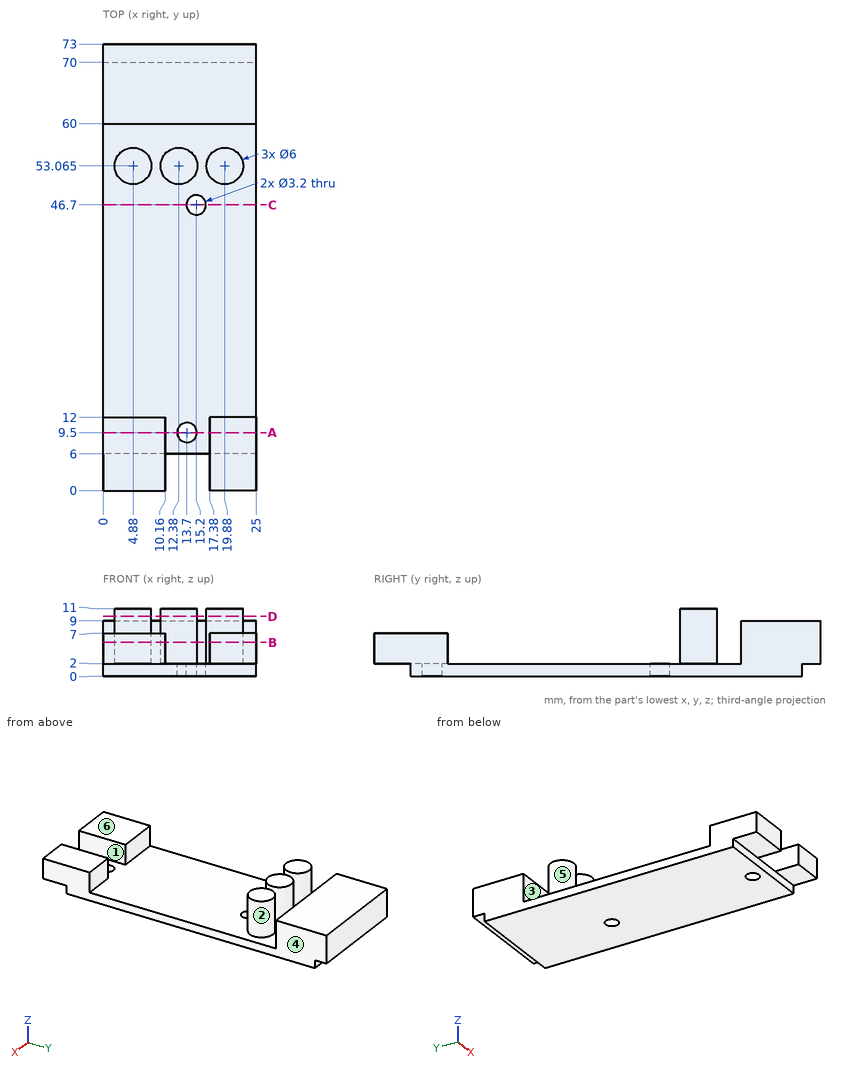
Study the drawing (mm; zero at the part's minimum x, y, z) and answer. A direction names the side the tool comes from. Give positions to 0.01 mm unless a question says otherwise; leave off trailing zeros. Write each loop counter-clockwise with the first axis right and the second up, starting at its lowest first coordinate (ties: lowest second). Pieces come first, ordered by that corner, then holes. Notation, with made-up numbers: (-26, -31) -> (0, -31) arc R19 cw to (0, -23) -> close; hole circle Ø7 at (75.25, 86). An arc over 180 degrees is marked (long way). Answer in a Markdown table with one row per item.
1) Each of these flat-tipped pins is pushed along its axis until it touches: pin 1 Ø1.5 at (x, z) = (12, 6) entering from -Y (1 decimal); pin 2 Ø3 at (x, z) = (3, 8) entering from -Y; pin 3 Ø1.5 at (x, z) = (18.5, 1) entering from -Y; pin 4 Ø2.5 at (x, y) = (21, 8) entering from +Z. Where does it stop, or does it pass through?
Results list:
| item | result |
|---|---|
| pin 1 | y = 50.1 |
| pin 2 | y = 0 |
| pin 3 | y = 6 |
| pin 4 | z = 7 |
2) Section D-D on z = 9.75 is taken. Give the vertices of the cut face in (x, y) (1 decimal).
Results list:
| item | result |
|---|---|
| outline | circle Ø6 at (4.9, 53.1); circle Ø6 at (12.4, 53.1); circle Ø6 at (19.9, 53.1) |
3) A tool of negligible diameter and unlimited length cuts with its end or side. For the marked faces 1, 2 and 3, from which of +Z, -Z, +X, -X, +Y, -Y can it reach the whole face along a straight path? Write none if from no direction.
Results list:
| item | result |
|---|---|
| face 1 | +Z, -Y |
| face 2 | +Z |
| face 3 | +Z, +X, -X |
4) Section B-B on z = 5.5 is taken. Give the vertices of the cut face in (x, y) (1 decimal), plus the area to 3 significant figures.
Results list:
| item | result |
|---|---|
| outline | (0, 0) -> (10.2, 0) -> (10.2, 12) -> (0, 12) -> close; (0, 60) -> (25, 60) -> (25, 73) -> (0, 73) -> close; circle Ø6 at (4.9, 53.1); circle Ø6 at (12.4, 53.1); circle Ø6 at (19.9, 53.1); (17.4, 0) -> (25, 0) -> (25, 12) -> (17.4, 12) -> close |
| area | 623 mm^2 |
5) Determine the mould class of the marked faces 4, 5 and 6 for opening direction X: released by +X, released by -X, zero draft, split by the parting line, or undercut.
Results list:
| item | result |
|---|---|
| face 4 | released by +X |
| face 5 | undercut |
| face 6 | zero draft |
6) Straight lines are drawn through the part: line 1 (Y direction, x = 22, z = 5.5); line 2 (Y direction, x = 23.5, z = 4.5); line 3 (X direction, y = 6.5, z = 6). For each, find the intervals that lie inside material, in ascending order. Write a range as [from, to].
Results list:
| item | result |
|---|---|
| line 1 | [0, 12], [50.94, 55.19], [60, 73] |
| line 2 | [0, 12], [60, 73] |
| line 3 | [0, 10.16], [17.38, 25] |
7) Section A-A on y = 9.5 is taken. Give the vertices of the cut face in (x, z).
Results list:
| item | result |
|---|---|
| outline | (0, 0) -> (12.1, 0) -> (12.1, 2) -> (10.16, 2) -> (10.16, 7) -> (0, 7) -> close; (15.3, 0) -> (25, 0) -> (25, 7) -> (17.38, 7) -> (17.38, 2) -> (15.3, 2) -> close |
8) Section C-C on y = 46.7 is taken. Give the vertices of the cut face in (x, z), plus the area to 3 significant figures.
Results list:
| item | result |
|---|---|
| outline | (0, 0) -> (13.6, 0) -> (13.6, 2) -> (0, 2) -> close; (16.8, 0) -> (25, 0) -> (25, 2) -> (16.8, 2) -> close |
| area | 43.6 mm^2 |
